Study the drawing (mm; zero at the part's minimum x, y, z) and answer. Coordinates: 2 decimals unless noted, no trailing zeros. Loops run counter-clockwise (first coordinate to the right, second up) from the corner with the lowest first, then second, coordinate; pieces in that order, holes last. Notation, with made-up numbers: (81, 48) -> (107, 48) arc R22 cw to (107, 63) -> close; hole circle Ø11 at (63, 63). An arc over 180 degrees is marked (long way). Answer as CSV lines item,"result".
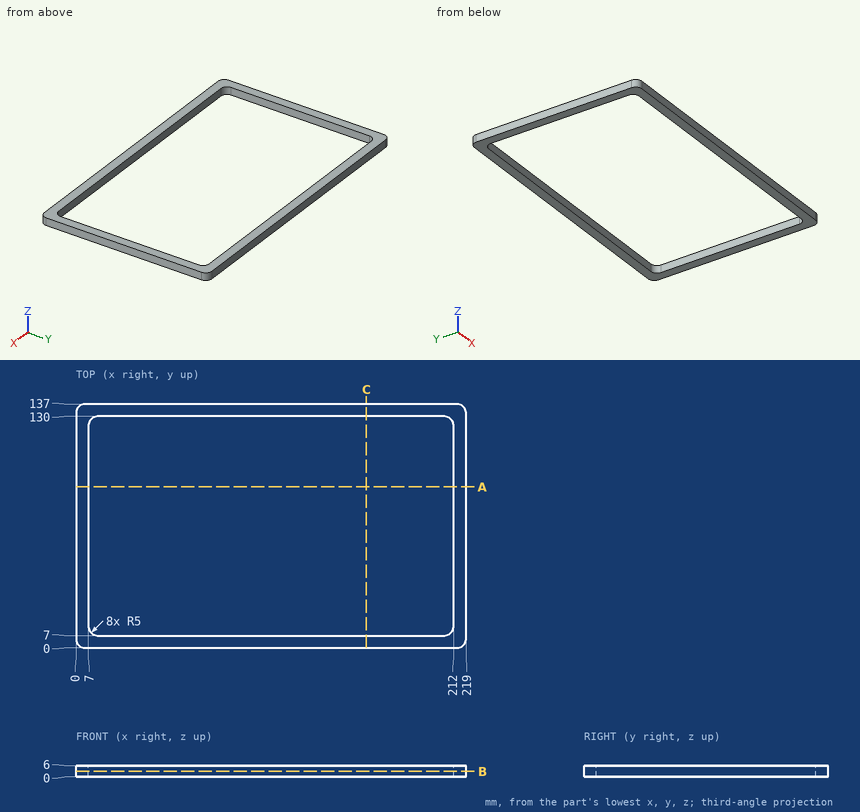
Q1. Find the intervals of material crossed by probe 1 along Y at (x, z) = (157.5, 1.35); probe 2 along X at (y, z) = (72.5, 2.85); probe 3 along X at (y, z) = (8.5, 0.65), in increasing order. Write a range as [from, to].
Results:
probe 1,"y = [0, 7], [130, 137]"
probe 2,"x = [0, 7], [212, 219]"
probe 3,"x = [0, 8.43], [210.57, 219]"
Q2. A cutting plane is placed at B-B, the plane z = 3. Write down the section's boundary in (x, y), and give its area (3 significant figures).
Results:
outline,"(0, 5) arc R5 ccw to (5, 0) -> (214, 0) arc R5 ccw to (219, 5) -> (219, 132) arc R5 ccw to (214, 137) -> (5, 137) arc R5 ccw to (0, 132) -> close; hole (7, 12) arc R5 ccw to (12, 7) -> (207, 7) arc R5 ccw to (212, 12) -> (212, 125) arc R5 ccw to (207, 130) -> (12, 130) arc R5 ccw to (7, 125) -> close"
area,"4,790 mm²"
Q3. A cutting plane is placed at C-C, the plane x = 163. Write down the section's boundary in (y, z), and give its area (3 significant figures).
Results:
outline,"(0, 0) -> (7, 0) -> (7, 6) -> (0, 6) -> close; (130, 0) -> (137, 0) -> (137, 6) -> (130, 6) -> close"
area,"84.0 mm²"
Q4. A cutting plane is placed at A-A, the plane y = 90.5. Write down the section's boundary in (x, z).
Results:
outline,"(0, 0) -> (7, 0) -> (7, 6) -> (0, 6) -> close; (212, 0) -> (219, 0) -> (219, 6) -> (212, 6) -> close"
